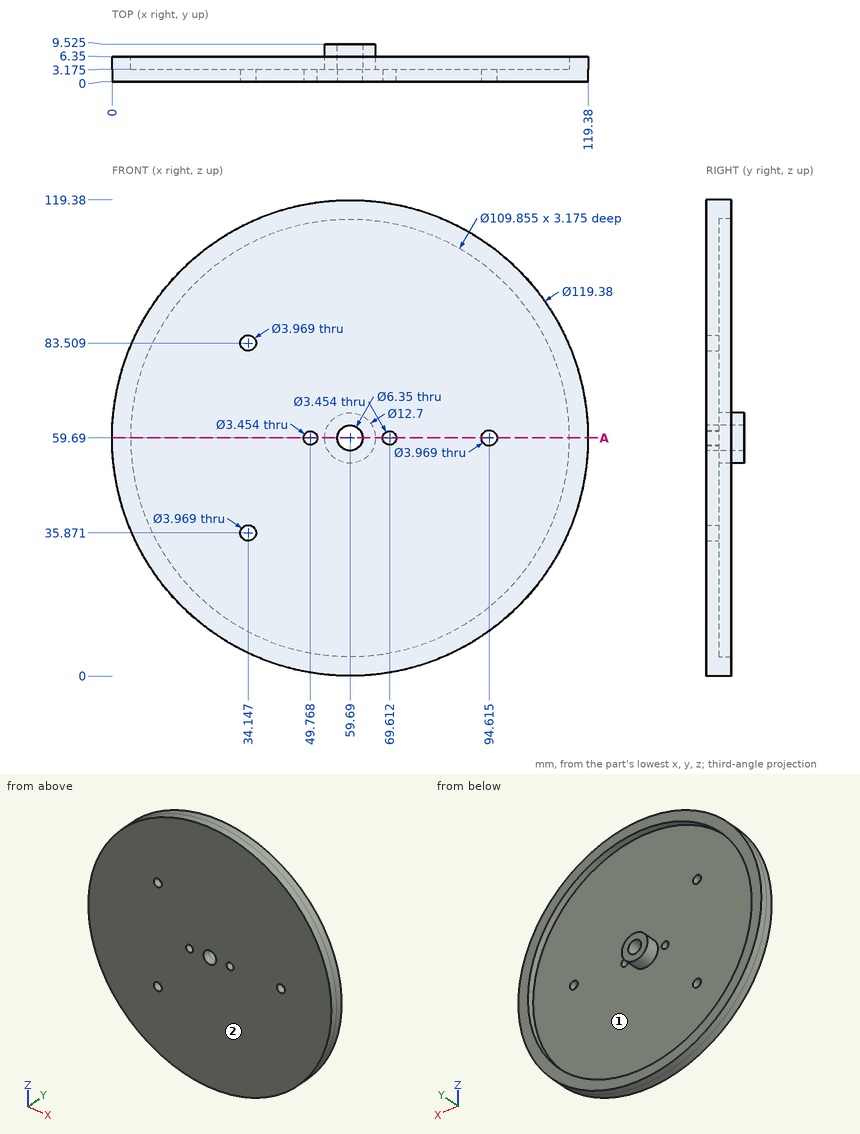
Answer from the drawing. Dimensions are ordinates in mm from the lowest x, y and z of the part. Round coordinates to 2 decimals unless told otherwise and drop trailing zeros. Write each question's results on one line, items separated by ' | '.
1) Flat-ended cylindrical pins translate along their axes: pin 1 (3.5 mm diameter, centred on x = 34.15, z = 35.87, fed in from +Y); pin 2 (1.5 mm diameter, centred on x = 54.5, y = 4.5, fed in from +Z) (1 decimal); pin 3 (1.5 mm diameter, centred on x = 83, y = 5.5, fed in from +Z); pin 4 (3 mm diameter, centred on y = 5.5, z = 106.5, fed in from -X). Find the tip coordinate at first contact, or state that the pin passes through.
Findings:
pin 1: passes through | pin 2: stops at z = 119.2 | pin 3: stops at z = 114.95 | pin 4: stops at x = 20.83
2) Consider line 1 along Z through (x, y) = (63, 4.75); line 2 along X through (y, z) = (3.5, 58) (1 decimal); line 3 along Y through (x, z) = (19, 73) (1 decimal). Determine where each line is inside the solid, lowest interval first. Write a range as [from, to].
Findings:
line 1: z = [0.09, 4.86], [54.27, 65.11], [114.52, 119.29] | line 2: x = [0, 4.8], [53.6, 57], [62.4, 65.8], [114.6, 119.4] | line 3: y = [0, 3.2]
3) For a pull along Z with two mould halves and no side action, classify the marked faces 1 and 2 as +Z half, -Z half, draft (parallel to the pull), parting line (faces both ways), or undercut.
Findings:
face 1: undercut | face 2: draft
4) The part is cut by section A-A (z = 59.69). State how many separate pieces and enclosed holes the cut face has, and give its area (3 significant figures).
Findings:
separate pieces: 5 | enclosed holes: 0 | area: 395 mm²
